```python
from build123d import *

# Parameters (mm, degrees)
SKETCH1_R               = 33
BOSS_EXTRUDE1_DEPTH     = 13
SKETCH2_R               = 13
BOSS_EXTRUDE2_DEPTH     = 3
CUT_EXTRUDE1_DEPTH      = 1
CUT_EXTRUDE1_DEPTH_BACK = 17


with BuildPart() as part:
    # Sketch1 → Boss-Extrude1 (new body)
    with BuildSketch(Plane(origin=(0, 0, 0), x_dir=(1, 0, 0), z_dir=(0, 1, 0))):
        Circle(SKETCH1_R)
    extrude(amount=BOSS_EXTRUDE1_DEPTH)

    # Sketch2 → Boss-Extrude2 (add)
    with BuildSketch(Plane(origin=(0, 13, 0), x_dir=(1, 0, 0), z_dir=(0, 1, 0))):
        Circle(SKETCH2_R)
    extrude(amount=BOSS_EXTRUDE2_DEPTH)

    # Sketch3 → Cut-Extrude1 (cut, two sides)
    with BuildSketch(Plane(origin=(0, 16, 0), x_dir=(1, 0, 0), z_dir=(0, 1, 0))) as cut_extrude1_sk:
        with BuildLine():
            ThreePointArc((2, 5.123475383), (0, 5.5), (-2, 5.123475383))
            Line((-2, 5.123475383), (-2, 5))
            Line((-2, 5), (2, 5))
            Line((2, 5), (2, 5.123475383))
        make_face()
        with BuildLine():
            Line((-2, 5), (-2, 5.123475383))
            ThreePointArc((-2, 5.123475383), (-3.102418411, -4.541475531), (5.5, 0))
            ThreePointArc((5.5, 0), (4.541475531, 3.102418411), (2, 5.123475383))
            Line((2, 5.123475383), (2, 5))
            Line((2, 5), (-2, 5))
        make_face()
        with BuildLine():
            Line((2, 6), (-2, 6))
            Line((-2, 6), (-2, 5.123475383))
            ThreePointArc((-2, 5.123475383), (0, 5.5), (2, 5.123475383))
            Line((2, 5.123475383), (2, 6))
        make_face()
    extrude(amount=CUT_EXTRUDE1_DEPTH, mode=Mode.SUBTRACT)
    extrude(cut_extrude1_sk.sketch, amount=-CUT_EXTRUDE1_DEPTH_BACK, mode=Mode.SUBTRACT)


solid = part.part
```
Design review of the part built by this model. Coordinates are the model's own, in mm. Round coordinates to 2 decimals unless told otherwise and drop trailing zeros. Write each loop counter-clockwise with the first axis right and the second up, starting at its lowest first coordinate (ties: lowest second). Pieces come first, ordered by that corner, then holes. Notation, with made-up numbers: (-38.75, 2.25) -> (6.25, 2.25) arc R22 ccw to (6.25, 30.25) -> close; hole circle Ø7 at (-28, 82). An arc over 180 degrees is marked (long way). Write item = value, one per line. Start each with the question number.
1) Take a section at A-A, the plane x = 0. State the section outline as (y, z) points, plus the area to 3 significant figures.
2) Mouldability with a two-part tool opening along X and no side actions: class faces 1 (the face through (0, 8, -6)), 2 (the face through (0, 13, 14)), 3 (the face through (-10.316, 14.479, 7.91)) as +X half, -X half, draft (parallel to the pull), parting line (faces both ways), or undercut.
3) Wall thickness on probe 1 along Z at (x, y) = (0, 7.5); probe 2 along Y at (x, z) = (1.5, -26.5); probe 3 along X at (y, z) = (0.75, 5): over which ranges is each line inside the solid? List them lowest first. Write a range as from..to.
4) Take a section at B-B, the plane z = 1. State the section outline as (x, y) points, plus the area to 3 significant figures.
5) Take a section at C-C, the plane y = 7. State the section outline as (x, z) points, plus the area to 3 significant figures.
6) Clearance check with flat-ended pins moving along their axes: pin 1 (8 mm diameter, centred on y = 5, z = 9, fed in from -X); pin 2 (1 mm diameter, centred on y = 10, z = -5.5, fed in from +X); pin 3 (1 mm diameter, centred on y = 11.5, z = -7, fed in from -X). State where each tip first meets the part, or that it passes through.
7) Take a section at D-D, the plane x = -8. State the section outline as (y, z) points, plus the area to 3 significant figures.
Results list:
q1.outline = (0, -33) -> (13, -33) -> (13, -13) -> (16, -13) -> (16, -6) -> (0, -6) -> close; (0, 5.5) -> (16, 5.5) -> (16, 13) -> (13, 13) -> (13, 33) -> (0, 33) -> close
q1.area = 752 mm²
q2.face_1 = undercut
q2.face_2 = draft
q2.face_3 = parting line
q3.probe_1 = -33..-6, 5.5..33
q3.probe_2 = 0..13
q3.probe_3 = -32.62..-2.29, 2.29..32.62
q4.outline = (-32.98, 0) -> (-5.41, 0) -> (-5.41, 16) -> (-12.96, 16) -> (-12.96, 13) -> (-32.98, 13) -> close; (5.41, 0) -> (32.98, 0) -> (32.98, 13) -> (12.96, 13) -> (12.96, 16) -> (5.41, 16) -> close
q4.area = 762 mm²
q5.outline = circle Ø66 at (0, 0); hole (-2, -6) -> (2, -6) -> (2, -5.12) arc R5.5 ccw (long way) to (-2, -5.12) -> close
q5.area = 3,320 mm²
q6.pin_1 = -32.62
q6.pin_2 = 32.62
q6.pin_3 = -32.35
q7.outline = (0, -32.02) -> (13, -32.02) -> (13, -10.25) -> (16, -10.25) -> (16, 10.25) -> (13, 10.25) -> (13, 32.02) -> (0, 32.02) -> close
q7.area = 894 mm²
